Build history of the part. All positions in model axes, mm. Face numbers are marked on the shaded views. A direction names the side the tool comes from. Round coordinates to 2 decimals unless told otherwise and drop trailing zeros. Write each loop counter-clockwise with the first axis right and the second up, starting at its lowest first coordinate (ties: lowest second). Pieces come first, ordered by that corner, then holes.
1) Flat gauge pins, fed straight in: pin 1 (3 mm diameter, centred on x = 43, y = 5, fed in from -Z); pin 2 (4 mm diameter, centred on y = 0, z = 67.5, fed in from -X); pin 3 (6 mm diameter, centred on x = -68, y = 3, fed in from +Z); pin 4 (4.5 mm diameter, centred on y = 0, z = 0, fed in from -X). Where does each tip first touch, or does it go through?
2) Saw through at A-A (z = 58.5). Write the cut outline in (x, y).
3) Wall check: probe 1 along X at (y, z) = (4, 17.5); probe 2 along Y at (x, z) = (-118.9, 0); probe 3 along Y at (x, z) = (24, 67.5). Give the ranges that are in metal, low to high.
4) Saw through at B-B (z = 0). Write the cut outline in (x, y).
5) Which spindle directions (+Z, -Z, +X, -X, +Y, -Y) get a long thin tool onto all of the face, cutting with end or side? Do the marked faces 4, 5, 6 and 7. Say none if no direction does.
6) Saw through at C-C (x = -43). Write the cut outline in (y, z), plus the area to 3 significant figures.
7) Pull direction X, two halves, no side cores. Call the marked faces 1, 2 and 3: +X half, -X half, draft (parallel to the pull), parting line (faces both ways), or undercut.
from build123d import *

# Parameters (mm, degrees)
BOSS_EXTRUDE1_DEPTH      = 10
BOSS_EXTRUDE1_DEPTH_BACK = 10
SKETCH2_R                = 2.5
CUT_EXTRUDE1_DEPTH       = 285
SKETCH3_R                = 1.7
SKETCH3_R_2              = 1.25
CUT_EXTRUDE2_DEPTH       = 285


with BuildPart() as part:
    # Sketch1 → Boss-Extrude1 (new body, two sides)
    with BuildSketch(Plane(origin=(0, 0, 0), x_dir=(1, 0, 0), z_dir=(0, 1, 0))) as boss_extrude1_sk:
        Polygon((-117.5, 10), (-119.5, 10), (-119.5, -20), (21.5, -20), (21.5, -80), (25.6, -80), (25.6, -20), (119.5, -20), (119.5, 10), (117.5, 10), (117.5, -18), (23.6, -18), (23.6, -78), (23.5, -78), (23.5, -18), (-117.5, -18), align=None)
    extrude(amount=BOSS_EXTRUDE1_DEPTH)
    extrude(boss_extrude1_sk.sketch, amount=-BOSS_EXTRUDE1_DEPTH_BACK)

    # Sketch2 → Cut-Extrude1 (cut)
    with BuildSketch(Plane.ZY.offset(119.5)):
        Circle(SKETCH2_R)
    extrude(amount=-CUT_EXTRUDE1_DEPTH, mode=Mode.SUBTRACT)

    # Sketch3 → Cut-Extrude2 (cut)
    with BuildSketch(Plane(origin=(25.6, 0, 0), x_dir=(0, 0, -1), z_dir=(1, 0, 0))):
        with Locations((-67.5, 0)):
            Circle(SKETCH3_R)
        with Locations((-72.449747468, -4.949747468)):
            Circle(SKETCH3_R_2)
        with Locations((-72.449747468, 4.949747468)):
            Circle(SKETCH3_R_2)
        with Locations((-62.550252532, 4.949747468)):
            Circle(SKETCH3_R_2)
        with Locations((-62.550252532, -4.949747468)):
            Circle(SKETCH3_R_2)
    extrude(amount=-CUT_EXTRUDE2_DEPTH, mode=Mode.SUBTRACT)


solid = part.part
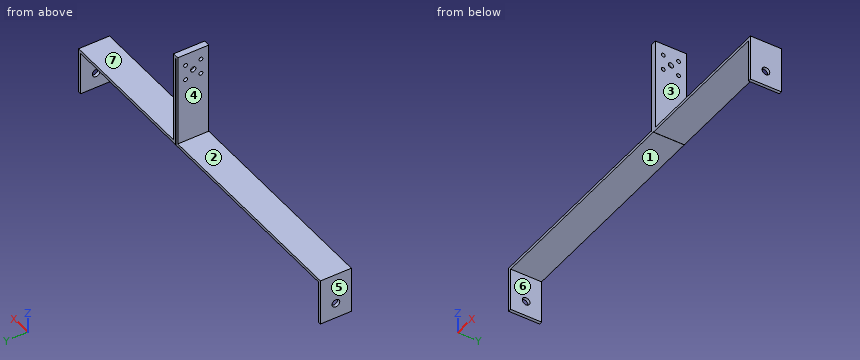
Evaluation:
1. pin 1: stops at z = 18
1. pin 2: stops at x = 21.5
1. pin 3: stops at z = 20
1. pin 4: passes through
2. outline: (21.5, -10) - (23.5, -10) - (23.5, 10) - (21.5, 10) - close; (23.6, -10) - (25.6, -10) - (25.6, 10) - (23.6, 10) - close
3. probe 1: x = -119.5 to -117.5, 117.5 to 119.5
3. probe 2: y = -10 to -2.5, 2.5 to 10
3. probe 3: y = -10 to -1.7, 1.7 to 10
4. outline: (-119.5, -10) - (-117.5, -10) - (-117.5, -2.5) - (-119.5, -2.5) - close; (-119.5, 2.5) - (-117.5, 2.5) - (-117.5, 10) - (-119.5, 10) - close; (117.5, -10) - (119.5, -10) - (119.5, -2.5) - (117.5, -2.5) - close; (117.5, 2.5) - (119.5, 2.5) - (119.5, 10) - (117.5, 10) - close
5. face 4: +Z, -X, +Y, -Y
5. face 5: +Z, -Z, -X, +Y, -Y
5. face 6: -Z, +Y, -Y
5. face 7: +Z, +X, +Y, -Y
6. outline: (-10, 18) - (10, 18) - (10, 20) - (-10, 20) - close
6. area: 40.0 mm2
7. face 1: undercut
7. face 2: draft
7. face 3: +X half
